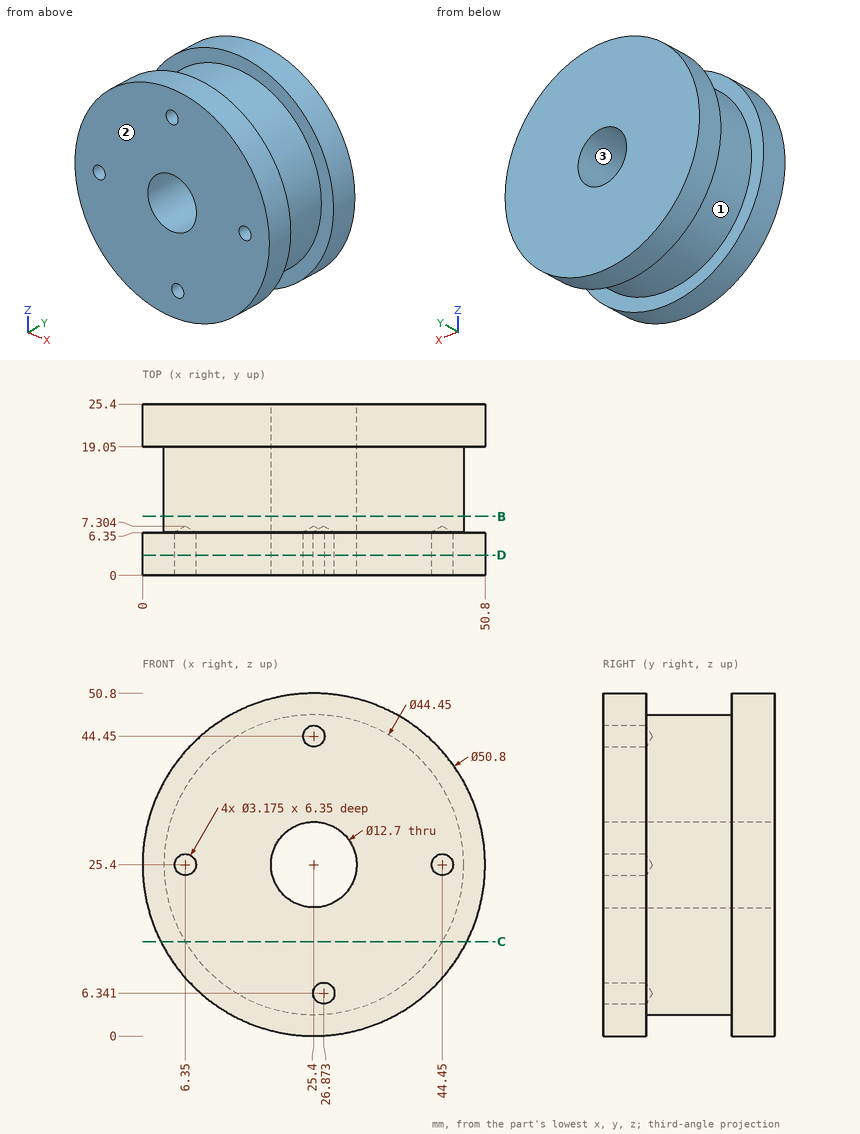
Answer from the drawing. Dimensions are ordinates in mm from the lowest x, y and z of the part. Coordinates: 2 decimals unless noted, no trailing zeros. Loops run counter-clockwise (first coordinate to the right, second up) from the corner with the lowest first, then second, coordinate; pieces in that order, holes last. Notation, with made-up numbers: (-2.75, 17.25) -> (47.25, 17.25) arc R24 cw to (47.25, 34.25) -> close; hole circle Ø3 at (1.25, 9). An arc over 180 degrees is marked (long way). Answer in a Markdown table with one row per item.
Item 1: Straight lines are drawn through the part: line 1 along Z through (x, y) = (25.4, 12.75) (3 decimals); line 2 along Y through (x, z) = (7.5, 10); line 3 along Z through (x, y) = (25, 22.75). For each, find the intervals that lie inside material, in ascending order. Write a range as [from, to].
Returned:
| item | result |
|---|---|
| line 1 | z = [3.175, 19.05], [31.75, 47.625] |
| line 2 | y = [0, 6.35], [19.05, 25.4] |
| line 3 | z = [0, 19.06], [31.74, 50.8] |
Item 2: For a pull along X with two mould halves and no side action, classify the marked faces 1, 2 and 3 as released by +X, released by -X, zero draft, split by the parting line, or undercut.
Returned:
| item | result |
|---|---|
| face 1 | split by the parting line |
| face 2 | zero draft |
| face 3 | undercut |
Item 3: A cutting plane is placed at B-B on y = 8.75. Determine the outline of the cut face in (x, z) (3 decimals).
Returned:
| item | result |
|---|---|
| outline | circle Ø44.45 at (25.4, 25.4); hole circle Ø12.7 at (25.4, 25.4) |
Item 4: Each of these flat-tipped pins is pushed along its axis until it touches: P1, Ø10, axis at x = 25.4, z = 25.4, coming from the -Y side; P2, Ø5, axis at x = 25.4, z = 44.45, coming from the -Y side; P3, Ø2, axis at y = 21, z = 43, coming from the -X side (1 decimal); P4, Ø4, axis at y = 18.5, z = 29.5, coming from the -X side. Where does it stop, or does it pass through?
Returned:
| item | result |
|---|---|
| P1 | passes through |
| P2 | stops at y = 0 |
| P3 | stops at x = 6.2 |
| P4 | stops at x = 0.09 |
Item 5: A cutting plane is placed at D-D on y = 3. Give the number of separate pieces and of enclosed holes in the cut face, plus the area to 3 significant figures.
Returned:
| item | result |
|---|---|
| separate pieces | 1 |
| enclosed holes | 5 |
| area | 1,870 mm^2 |
Item 6: A cutting plane is placed at C-C on z = 14. Determine the outline of the cut face in (x, y).
Returned:
| item | result |
|---|---|
| outline | (2.7, 0) -> (48.1, 0) -> (48.1, 6.35) -> (44.48, 6.35) -> (44.48, 19.05) -> (48.1, 19.05) -> (48.1, 25.4) -> (2.7, 25.4) -> (2.7, 19.05) -> (6.32, 19.05) -> (6.32, 6.35) -> (2.7, 6.35) -> close |
